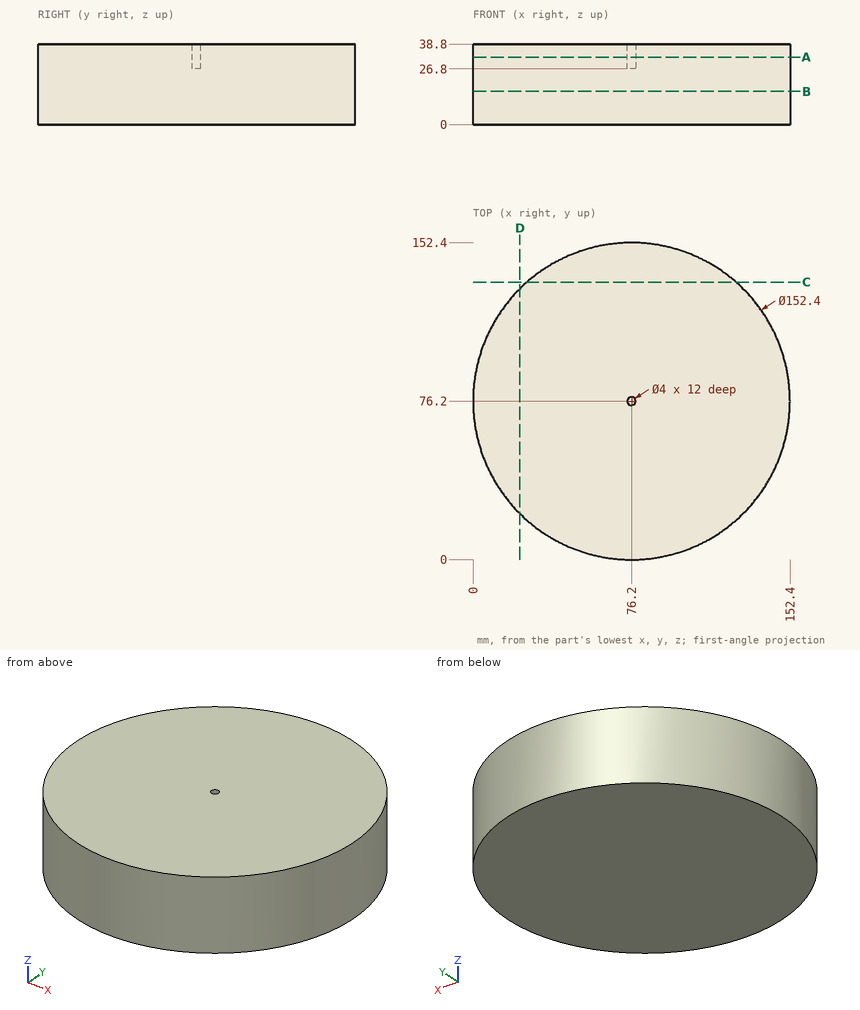
Part print with two shaded views. Sizes in mm from the minimum x, y, z corner. Round coordinates to 2 decimals unless told otherwise and drop trailing zeros. Order: outer loops, then holes, each group sorted by start corner. A loop starts at its lowest first (then second) coordinate and runs counter-clockwise, first axis right, second up. Notation, with made-up numbers: (-28, 26) - (29, 26) arc R24 cw to (29, 62) - close; hole circle Ø11 at (61.5, -21). An arc over 180 degrees is marked (long way). Answer in a Markdown table with one row per item. Add a question column.
(1) Drop flat-ended pins along their axis: pin 1 Ø1 at (x, z) = (134.5, 34.5) entering from -Y; pin 2 Ø12 at (x, z) = (124.5, 11) entering from -Y; pin 3 Ø1.5 at (x, z) = (118, 21.5) entering from +Y. Give the stop position or say it passes through.
(2) Band-saw the part on B-B on z = 16. List the corners of the cut face in (x, y), and give its area (3 significant figures).
(3) Band-saw the part on D-D on x = 22.5. List the corners of the cut face in (y, z).
(4) Band-saw the part on C-C on y = 133.5. List the corners of the cut face in (x, z), and give its area (3 significant figures).
(5) Band-saw the part on A-A on z = 32.5. List the corners of the cut face in (x, y).
(6) Probe L1, parallel to Y at x = 76, z = 35; L2, parallel to X at y = 78, z = 8.5. List the from-to ranges inside material, lowest first. Write a range as [from, to].
Data:
| question | item | result |
|---|---|---|
| 1 | pin 1 | stops at y = 26.55 |
| 1 | pin 2 | stops at y = 12.82 |
| 1 | pin 3 | stops at y = 140.4 |
| 2 | outline | circle Ø152.4 at (76.2, 76.2) |
| 2 | area | 18,200 mm^2 |
| 3 | outline | (22.14, 0) - (130.26, 0) - (130.26, 38.8) - (22.14, 38.8) - close |
| 4 | outline | (25.97, 0) - (126.43, 0) - (126.43, 38.8) - (25.97, 38.8) - close |
| 4 | area | 3,900 mm^2 |
| 5 | outline | circle Ø152.4 at (76.2, 76.2); hole circle Ø4 at (76.2, 76.2) |
| 6 | L1 | y = [0, 74.21], [78.19, 152.4] |
| 6 | L2 | x = [0.02, 152.38] |
